Check sheet for the modelled part. Datum: model origin and axes. Units: mm. Face numbers are marked on the shaded views. A direction names the side the tool comes from. Round coordinates to 2 decimals unless told otherwise and drop trailing zeros. Loops run counter-clockwise (first coordinate to the right, second up) from the corner with the lowest first, then second, coordinate; pieces in that order, holes last. Notation, with made-up numbers: M 24.25,67.25 L 40.25,67.25 A22 ccw 40.25,85.25 Z; hole C -11,-35 d9. An arc over 180 degrees is marked long. One line per question, with ' | ' between items. Start each with the question number.
(1) Go/stop test with flat-tipped pins: P1, Ø3, axis at y = 2.5, z = -0.5, coming from the +X side; P2, Ø1.5, axis at y = 2, z = -1, coming from the +X side; P3, Ø1.5, axis at y = 2.5, z = 0, coming from the +X side. Record where each tip stops, or that it passes through.
(2) Thickness scan on probe 1 along Z at (x, y) = (2, 3.2); probe 2 along Y at (x, z) = (2.5, -0.5); probe 3 along Z at (x, y) = (-0.5, 1.1). Record the ranges inside material, lowest first. Write a range as [from, to].
(3) Section check B-B (z = 0). Record the boundary of the cut face in (x, y) (3 decimals).
(4) Section check C-C (y = 2.15). Record the boundary of the cut face in (x, z).
(5) Tool access check on the marked faces 1 and 2. Record the directions out of +Z, -Z, +X, -X, +Y, -Y that give a thin tool (end or side, any length) a straight path to the whole face; none if there is none.
(6) Draft check along X on the marked faces 3, 4 and 5. Enter one of: +X half, -X half, draft (parallel to the pull), parting line (faces both ways), or undercut.
(7) Section check A-A (y = 1.2). Record the boundary of the cut face in (x, z).
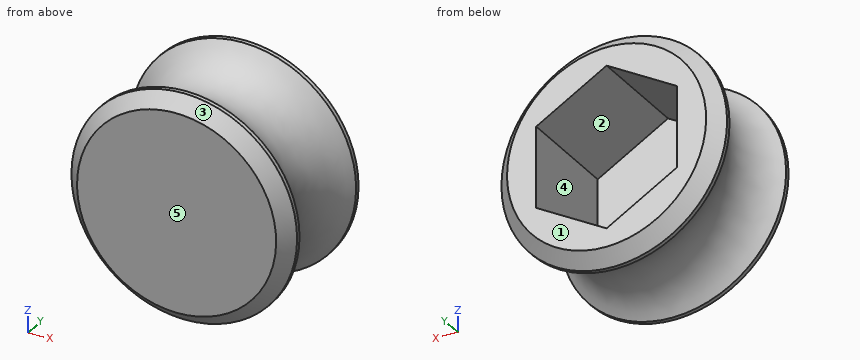
Autodesk Inventor part; units mm, degrees
ref_plane "Work Plane1" through (0, 2.5, 0) normal (0, 1, 0) x (1, 0, 0)
ref_plane "YZ Plane" through (0, 0, 0) normal (1, 0, 0) x (0, 1, 0)
ref_plane "XZ Plane" through (0, 0, 0) normal (0, 1, 0) x (-1, 0, 0)
sketch "Sketch1" plane through (0, 0, 0) normal (0, 1, 0) x (-1, 0, 0)
  line L0 (2.65, -1.53) -> (0, -3.06)
  line L1 (0, -3.06) -> (-2.65, -1.53)
  line L2 (-2.65, -1.53) -> (-2.65, 1.53)
  line L3 (-2.65, 1.53) -> (0, 3.06)
  line L4 (0, 3.06) -> (2.65, 1.53)
  line L5 (2.65, 1.53) -> (2.65, -1.53)
  circle A0 centre (0, 0) radius 3.5
  dimension "d1" = 5.3
  dimension "d2" = 7
extrude "Extrusion1" add sketch "Sketch1" along normal blind 5
sketch "Sketch2" plane through (0, 0, 0) normal (1, 0, 0) x (0, 1, 0)
  line L0 (0, -3.5) -> (5, -3.5)
  circle A0 centre (2.5, -5.75) radius 2.375
  line L1 (5, -3.5) -> (5, 3.5)
  line L2 (5, -3.5) -> (5, -4.25)
  line L3 (5, -4.25) -> (4.3414, -4.25)
  line L4 (0, -3.5) -> (0, 3.5)
  line L5 (0, -3.5) -> (0, -4.25)
  line L6 (0, -4.25) -> (0.6586, -4.25)
  line L7 (-1, 0) -> (6, 0)
  point P0 (0, 0)
  point P1 (1.7397, -3.5)
  point P2 (3.2603, -3.5)
  dimension "d5" = 4.75
  dimension "d6" = 2.25
  dimension "d7" = 0.75
  dimension "d8" = 0.75
revolve "Revolution1" cut sketch "Sketch2" angle 360 about axis through (0, -10, 0) along (0, 1, 0) contours A0 L0 | L0 A0
revolve "Revolution2" add sketch "Sketch2" angle 360 about axis through (0, -10, 0) along (0, 1, 0) contours L0 A0 L6 L5 | L0 L2 L3 A0
chamfer "Chamfer1" distance 0.5 angle 45 2 edges at (0, 5, 4.25) (0, 0, 4.25)
ref_plane "Work Plane1" through (0, 2.5, 0) normal (0, 1, 0) x (1, 0, 0)
sketch "Sketch3" plane through (0, 0, 0) normal (0, -1, 0) x (1, 0, 0)
  line L0 (-2.65, -1.53) -> (0, -3.06)
  line L1 (-2.65, 1.53) -> (-2.65, -1.53)
  line L2 (0, 3.06) -> (-2.65, 1.53)
  line L3 (2.65, 1.53) -> (0, 3.06)
  line L4 (2.65, -1.53) -> (2.65, 1.53)
  line L5 (0, -3.06) -> (2.65, -1.53)
  circle A0 centre (0, 0) radius 3.75
extrude "Extrusion2" add sketch "Sketch3" against normal blind 1 contours L1 L2 L3 L4 L5 L0
properties part number "5mm Hex Bearing Inside Blocker"
The answers:
1) P1: x = 3.89 | P2: x = 3.63 | P3: x = 3.5
2) probe 1: [-2.85, -1.91], [1.91, 2.85] | probe 2: [0, 1] | probe 3: [-3.8, -2.77], [2.77, 3.8]
3) outline: M -4.25,0.5 L -3.75,0 L 3.75,0 L 4.25,0.5 L 4.25,0.659 A2.375 cw 4.25,4.341 L 4.25,4.5 L 3.75,5 L 2.65,5 L 2.65,1 L -2.65,1 L -2.65,5 L -3.75,5 L -4.25,4.5 L -4.25,4.341 A2.375 cw -4.25,0.659 Z
4) outline: C 0,0 d6.8; hole M -2.65,-1.53 L 0,-3.06 L 2.65,-1.53 L 2.65,1.53 L 0,3.06 L -2.65,1.53 Z
5) face 1: +Z, -Z, +X, -X, +Y | face 2: +Y
6) face 3: parting line | face 4: undercut | face 5: draft
7) outline: C 0,0 d7.52; hole M -2.65,-1.53 L 0,-3.06 L 2.65,-1.53 L 2.65,1.53 L 0,3.06 L -2.65,1.53 Z
